Part print with two shaded views. Sizes in mm from the minimum x, y, z corner. Round coordinates to 2 decimals unless told otherwise and drop trailing zeros. Order: outer loops, then holes, each group sorted by start corner. A loop starts at its lowest first (then second) coordinate and runs counter-clockwise, first axis right, second up. Notation, with made-up numbers: M -18,49.25 L -9,49.25 A36 cw -9,86.25 Z; hole C -31,56 d3. An arc over 180 degrees is marked long. Answer as a JSON object with one key per item and string values.
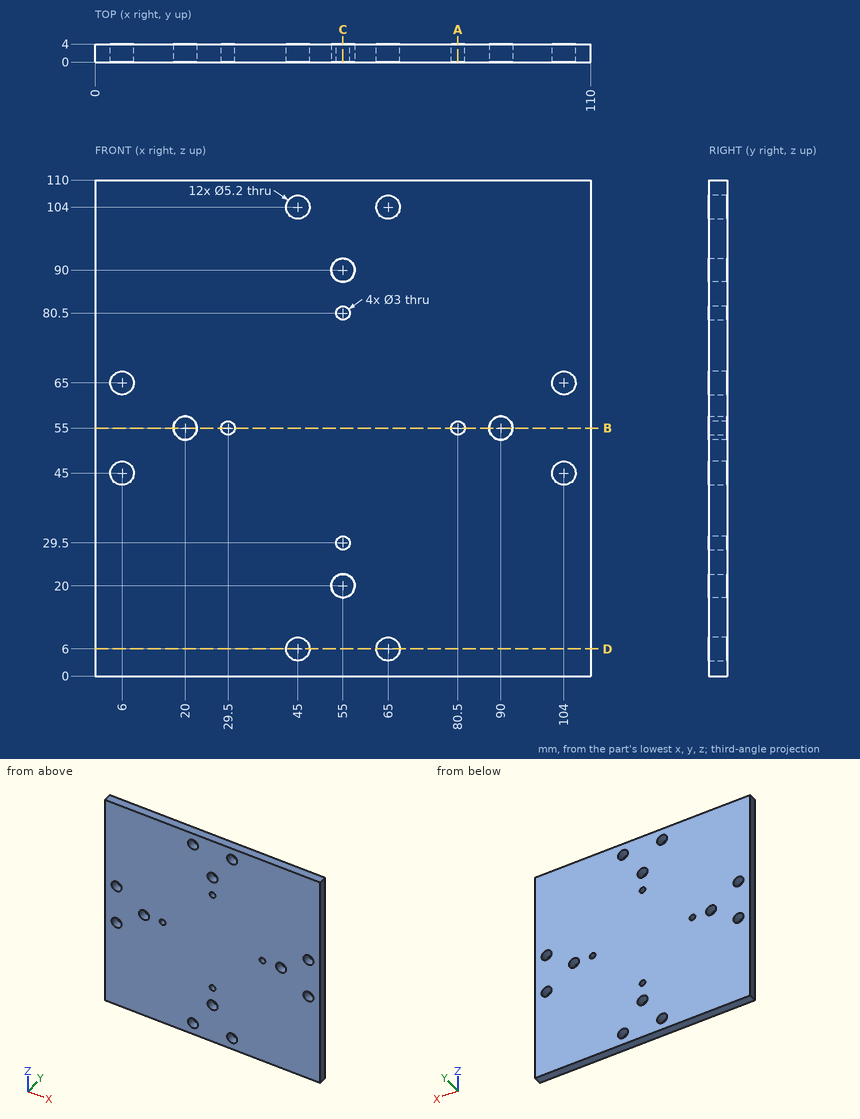
Item 1: Saw through at D-D on z = 6. List the corners of the cut face in (x, y), and give its area (3 significant figures).
Worked answers:
{"outline": "M 0,0 L 42.4,0 L 42.4,4 L 0,4 Z; M 47.6,0 L 62.4,0 L 62.4,4 L 47.6,4 Z; M 67.6,0 L 110,0 L 110,4 L 67.6,4 Z", "area": "398 mm2"}
Item 2: Wall check: line 1 along X through (y, z) = (1.55, 45); line 2 along Z through (x, y) = (53, 1); line 3 along X through (y, z) = (2.5, 55). Give the ranges that are in metal, low to high. Write a range as [from, to].
Worked answers:
{"line 1": "x = [0, 3.4], [8.6, 101.4], [106.6, 110]", "line 2": "z = [0, 18.34], [21.66, 88.34], [91.66, 110]", "line 3": "x = [0, 17.4], [22.6, 28], [31, 79], [82, 87.4], [92.6, 110]"}
Item 3: Saw through at A-A on x = 80.5. List the corners of the cut face in (y, z).
Worked answers:
{"outline": "M 0,0 L 4,0 L 4,53.5 L 0,53.5 Z; M 0,56.5 L 4,56.5 L 4,110 L 0,110 Z"}
Item 4: Saw through at C-C on x = 55. List the corners of the cut face in (y, z), and give its area (3 significant figures).
Worked answers:
{"outline": "M 0,0 L 4,0 L 4,17.4 L 0,17.4 Z; M 0,22.6 L 4,22.6 L 4,28 L 0,28 Z; M 0,31 L 4,31 L 4,79 L 0,79 Z; M 0,82 L 4,82 L 4,87.4 L 0,87.4 Z; M 0,92.6 L 4,92.6 L 4,110 L 0,110 Z", "area": "374 mm2"}
Item 5: Saw through at B-B on z = 55. List the corners of the cut face in (x, y).
Worked answers:
{"outline": "M 0,0 L 17.4,0 L 17.4,4 L 0,4 Z; M 22.6,0 L 28,0 L 28,4 L 22.6,4 Z; M 31,0 L 79,0 L 79,4 L 31,4 Z; M 82,0 L 87.4,0 L 87.4,4 L 82,4 Z; M 92.6,0 L 110,0 L 110,4 L 92.6,4 Z"}
